Can you work these out from the model? Positions are in its coordinate system, mm. Face numbers are marked on the shaded views. Give positions to 0.01 mm unless a question says otherwise; leave off trailing zeros. Write each loop counter-clockwise with the first axis right and the second up, starting at its lowest first coordinate (ties: lowest second). Pieces come first, ordered by that corner, then holes.
from build123d import *

# Parameters (mm, degrees)
F0_W     = 21.59
F0_H     = 27.94
F1_DEPTH = 9.525
F2_SIZE2 = 2.54
F2_SIZE  = 2.54
F3_R     = 3.302
F4_DEPTH = 9.526
F6_D     = 6.8


with BuildPart() as f1:
    # F0 (on Top) → F1 (new body)
    with BuildSketch(Plane.XY):
        Rectangle(F0_W, F0_H)
    extrude(amount=F1_DEPTH)

    # F2
    f2_edges = [f1.edges().sort_by_distance(p)[0] for p in [
        (-10.795, 13.97, 4.7625),
        (-10.795, -13.97, 4.7625),
        (10.795, -13.97, 4.7625),
        (10.795, 13.97, 4.7625),
    ]]
    chamfer(f2_edges, length=F2_SIZE, length2=F2_SIZE2)

    # F3 (on face) → F4 (cut, through all)
    with BuildSketch(Plane.XY.offset(9.525)):
        Circle(F3_R)
    extrude(amount=-F4_DEPTH, mode=Mode.SUBTRACT)

    # F6 (through all)
    with Locations(Plane.XY.offset(9.525)):
        with Locations((0, 0)):
            Hole(F6_D / 2)


solid = f1.part
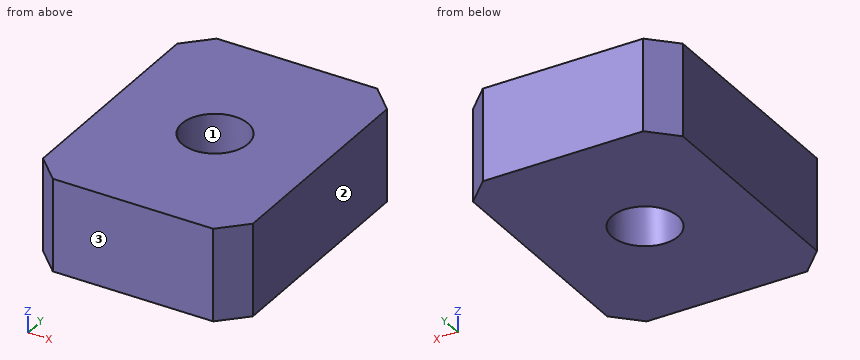
(1) Imagine slicing it at A-A, the plane y = 0. Write out the boundary of the cut face in (x, z) (3 decimals).
Returned:
outline: (-10.795, 0) - (-3.4, 0) - (-3.4, 9.525) - (-10.795, 9.525) - close; (3.4, 0) - (10.795, 0) - (10.795, 9.525) - (3.4, 9.525) - close
(2) If I drill on L1, parallel to Y at x = 0, z = 2.5; L2, parallel to X at y = -2.5, z = 2.75 (3 decimals); L3, parallel to Y at x = 2.5, z = 5.25, over which ranges is the centre line in solid material (lowest first)?
Returned:
L1: y = -13.97 to -3.4, 3.4 to 13.97
L2: x = -10.795 to -2.304, 2.304 to 10.795
L3: y = -13.97 to -2.3, 2.3 to 13.97
(3) If we mould it in two halves opening along Y, with no side actions, what happens to the marked faces 1, 2 and 3? For each: +Y half, -Y half, draft (parallel to the pull), parting line (faces both ways), or undercut.
Returned:
face 1: undercut
face 2: draft
face 3: -Y half
(4) Imagine slicing it at B-B, the plane x = 0. Write out the boundary of the cut face in (y, z) (3 decimals), plus the area to 3 significant figures.
Returned:
outline: (-13.97, 0) - (-3.4, 0) - (-3.4, 9.525) - (-13.97, 9.525) - close; (3.4, 0) - (13.97, 0) - (13.97, 9.525) - (3.4, 9.525) - close
area: 201 mm2
(5) Imagine slicing it at C-C, the plane z = 2.5. Write out the boundary of the cut face in (x, y) (3 decimals).
Returned:
outline: (-10.795, -11.43) - (-8.255, -13.97) - (8.255, -13.97) - (10.795, -11.43) - (10.795, 11.43) - (8.255, 13.97) - (-8.255, 13.97) - (-10.795, 11.43) - close; hole circle Ø6.8 at (0, 0)
